Design review of the part built by this model. Coordinates are the model's own, in mm. Coordinates: 2 decimals unless noted, no trailing zeros. Order: outer loops, then holes, each group sorted by start corner. A loop starts at its lowest first (then second) coordinate and runs counter-clockwise, first axis right, second up. Notation, with made-up numbers: (-20, -28) -> (3, -28) arc R22 cw to (3, -20) -> close; hole circle Ø11 at (-34.75, -12). An arc over 180 degrees is marked (long way). Use a Markdown table: item, result. Add a question column.
Q1. Insertion check: pin 1 (5 mm diameter, centred on y = 12.7, z = 311.15, fed in from -X). The pin has a flat end and moves straight along its axis. Give the tip position at first contact, or say it passes through.
Q2. Add section C-C (y = 12.7). Count the separate pieces of the cut face and the enclosed holes in it, then the cut area to 3 significant figures.
Q3. Add section B-B (x = 39). State the section outline as (y, z) points (3 decimals), then the cut area to 3 significant figures.
Q4. Add section A-A (z = 311.15). State the section outline as (x, y) points (3 decimals), then the cut area to 3 significant figures.
Q5. Wall thickness on probe 1 along X at (y, z) = (8, 115) (3 decimals); probe 2 along Y at (x, z) = (23, 334.5) (3 decimals); probe 3 along Y at (x, z) = (49, 311): over which ranges is each line inside the solid? List them lowest first.
Q6. Add section D-D (z = 106). State the section outline as (x, y) points (3 decimals), then the cut area to 3 significant figures.
from build123d import *

# Parameters (mm, degrees)
SKETCH1_W               = 50.8
SKETCH1_H               = 25.4
SKETCH1_W_2             = 44.45
SKETCH1_H_2             = 19.05
BOSS_EXTRUDE1_DEPTH     = 355.6
CUT_EXTRUDE1_DEPTH      = 361.10715072
CUT_EXTRUDE1_DEPTH_BACK = 361.10715072
SKETCH2_R               = 3.175


with BuildPart() as part:
    # Sketch1 → Boss-Extrude1 (new body)
    with BuildSketch(Plane.XY):
        with Locations((25.4, 12.7)):
            Rectangle(SKETCH1_W, SKETCH1_H)
        with Locations((25.4, 12.7)):
            Rectangle(SKETCH1_W_2, SKETCH1_H_2, mode=Mode.SUBTRACT)
    extrude(amount=BOSS_EXTRUDE1_DEPTH)

    # Sketch2 → Cut-Extrude1 (cut, two sides: drawn at the far end of the back side and taken through both)
    with BuildSketch(Plane(origin=(50.8, 0, 0), x_dir=(0, 0, -1), z_dir=(1, 0, 0)).offset(-CUT_EXTRUDE1_DEPTH_BACK)):
        with Locations((-273.05, 12.7)):
            Circle(SKETCH2_R)
        with Locations((-311.15, 12.7)):
            Circle(SKETCH2_R)
        with Locations(Location((-44.45, 12.7, 0), (0, 0, 180))):
            Circle(SKETCH2_R)
        with Locations(Location((-82.55, 12.7, 0), (0, 0, 180))):
            Circle(SKETCH2_R)
    extrude(amount=CUT_EXTRUDE1_DEPTH + CUT_EXTRUDE1_DEPTH_BACK, mode=Mode.SUBTRACT)


solid = part.part
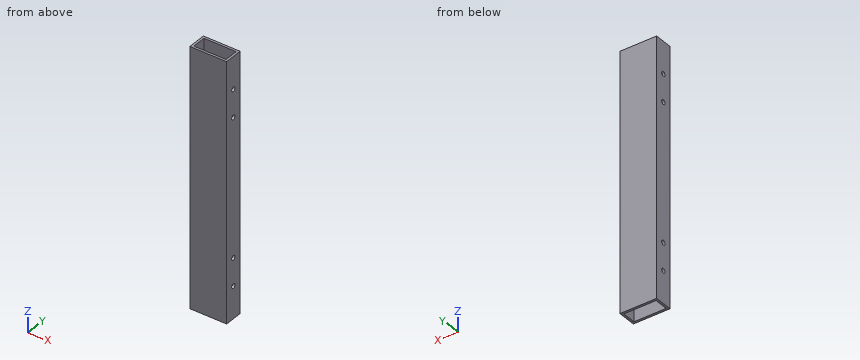
Established:
| question | item | result |
|---|---|---|
| 1 | pin 1 | through |
| 2 | separate pieces | 10 |
| 2 | enclosed holes | 0 |
| 2 | area | 2,100 mm^2 |
| 3 | outline | (0, 0) -> (3.175, 0) -> (3.175, 355.6) -> (0, 355.6) -> close; (22.225, 0) -> (25.4, 0) -> (25.4, 355.6) -> (22.225, 355.6) -> close |
| 3 | area | 2,260 mm^2 |
| 4 | outline | (0, 0) -> (50.8, 0) -> (50.8, 9.525) -> (47.625, 9.525) -> (47.625, 3.175) -> (3.175, 3.175) -> (3.175, 9.525) -> (0, 9.525) -> close; (0, 15.875) -> (3.175, 15.875) -> (3.175, 22.225) -> (47.625, 22.225) -> (47.625, 15.875) -> (50.8, 15.875) -> (50.8, 25.4) -> (0, 25.4) -> close |
| 4 | area | 403 mm^2 |
| 5 | probe 1 | 0 to 3.175, 47.625 to 50.8 |
| 5 | probe 2 | 0 to 3.175, 22.225 to 25.4 |
| 5 | probe 3 | 0 to 9.53, 15.87 to 25.4 |
| 6 | outline | (0, 0) -> (50.8, 0) -> (50.8, 25.4) -> (0, 25.4) -> close; hole (3.175, 3.175) -> (47.625, 3.175) -> (47.625, 22.225) -> (3.175, 22.225) -> close |
| 6 | area | 444 mm^2 |
